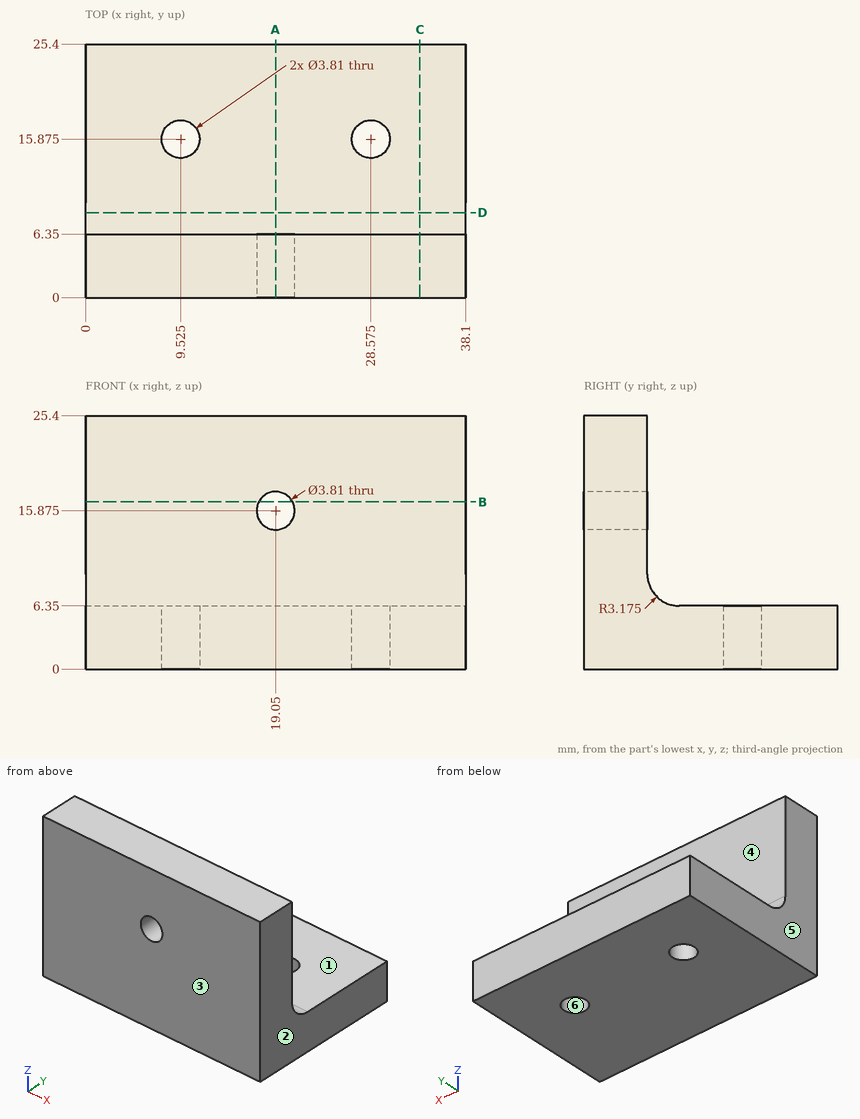
Print and shaded views of the part. All mm, measured from the part's lowest x, y and z. A direction names the side the tool comes from. Coordinates: 2 decimals unless noted, no trailing zeros. Write each loop counter-clockwise with the first axis right and the second up, starting at its lowest first coordinate (ties: lowest second). Pieces come first, ordered by that corner, then holes.
(1) Flat gauge pins, fed straight in: pin 1 (6 mm diameter, centred on x = 15, z = 20.5, fed in from +Y); pin 2 (5 mm diameter, centred on x = 33.5, y = 15.5, fed in from +Z). Where does each tip first touch, or does it go through?
(2) Two-plate mould, pull along Y, no slides. Class the marked faces 3, 4, 5 and 6: +Y half, -Y half, draft (parallel to the pull), parting line (faces both ways), or undercut.
(3) Drill centre lines: probe 1 along X at (y, z) = (4.25, 16); probe 2 along Z at (x, y) = (19.05, 4); probe 3 along Y at (x, z) = (3, 18.5). Where is each one in solid material? Low to high.
(4) Cut at C-C, the plane x = 33.5. List the corners of the cut face in (y, z) (3 decimals).
(5) Cut at B-B, the plane z = 16.75. List the corners of the cut face in (x, y).
(6) 3-axis set-ups, long thin cutter, end or side, ignore diameter. For the marked faces 1 and 2: which of +Z, -Z, +X, -X, +Y, -Y reach the whole face in a straight line?
(7) Cut at D-D, the plane y = 8.5. List the corners of the cut face in (x, z), and give its area (3 significant figures).
(8) Cut at A-A, the plane x = 19.05. List the corners of the cut face in (y, z) (3 decimals), and give its area (3 significant figures).
Geometry says:
1. pin 1: stops at y = 6.35
1. pin 2: stops at z = 6.35
2. face 3: -Y half
2. face 4: +Y half
2. face 5: draft
2. face 6: undercut
3. probe 1: x = 0 to 17.15, 20.95 to 38.1
3. probe 2: z = 0 to 13.97, 17.78 to 25.4
3. probe 3: y = 0 to 6.35
4. outline: (0, 0) - (25.4, 0) - (25.4, 6.35) - (9.525, 6.35) arc R3.175 cw to (6.35, 9.525) - (6.35, 25.4) - (0, 25.4) - close
5. outline: (0, 0) - (17.36, 0) - (17.36, 6.35) - (0, 6.35) - close; (20.74, 0) - (38.1, 0) - (38.1, 6.35) - (20.74, 6.35) - close
6. face 1: +Z, +X, -X, +Y
6. face 2: +Z, -Z, +X, +Y, -Y
7. outline: (0, 0) - (38.1, 0) - (38.1, 6.52) - (0, 6.52) - close
7. area: 248 mm2
8. outline: (0, 0) - (25.4, 0) - (25.4, 6.35) - (9.525, 6.35) arc R3.175 cw to (6.35, 9.525) - (6.35, 13.97) - (0, 13.97) - close; (0, 17.78) - (6.35, 17.78) - (6.35, 25.4) - (0, 25.4) - close
8. area: 260 mm2
